Can you work these out from the drawing? Everything is in mm from the part's minimum corner. A direction names the side the tool comes from. Coordinates: 2 decimals unless noted, no trailing zeros. Write each loop counter-clockwise with the first axis right and the second up, starting at its lowest first coordinate (ties: lowest second). Pieces come first, ordered by that corner, then holes. Notation, with made-up numbers: M 13,32.25 L 67,32.25 A27 cw 67,66.25 Z; hole C -13,39 d8. An arc over 180 degrees is marked long. Write item = value, one per line.
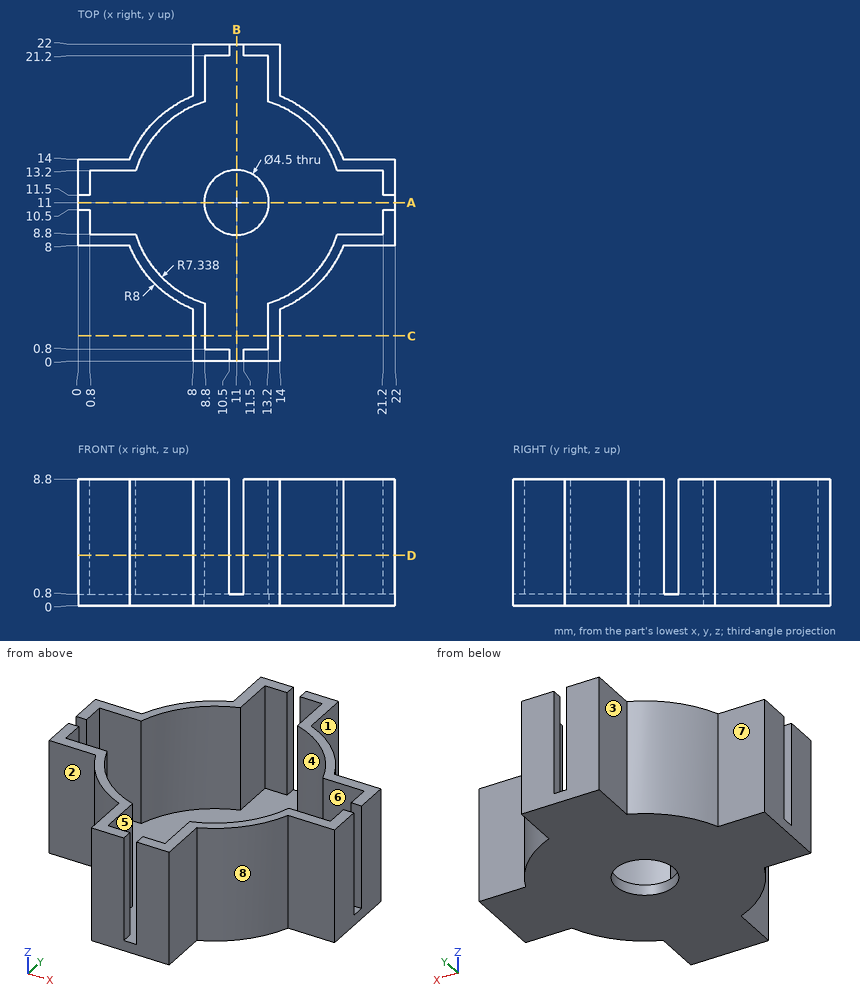
Item 1: I'm going to push flat-ended pins straight in: P1, Ø3.5, axis at y = 19, z = 6, coming from the +X side (1 decimal); P2, Ø1.6, axis at x = 1.5, z = 3, coming from the +Y side; P3, Ø1, axis at x = 3.5, z = 6, coming from the -Y side (1 decimal); P4, Ø1.4, axis at x = 9.5, z = 6, coming from the -Y side. Where does each tip first touch, or does it pass through?
Numbers:
P1 = 16
P2 = 14
P3 = 7.1
P4 = 0
Item 2: Imagine slicing it at D-D (z = 3.5). State how many separate pieces and enclosed holes the cut face has.
Numbers:
separate_pieces = 4
enclosed_holes = 0
Item 3: If I drill on line 1 along X through (y, z) = (18.5, 7); line 2 along Y through (x, z) = (11, 0.2), over which ranges is the centre line in solid material (lowest first)?
Numbers:
line_1 = 8 to 8.8, 13.2 to 14
line_2 = 0 to 8.75, 13.25 to 22
Item 4: Imagine slicing it at C-C (y = 1.75). Write out the boundary of the cut face in (x, z).
Numbers:
outline = M 8,0 L 14,0 L 14,8.8 L 13.2,8.8 L 13.2,0.8 L 8.8,0.8 L 8.8,8.8 L 8,8.8 Z
Item 5: For the marked faces 1, 2, 3 and 4, which set-ups out of +Z, -Z, +X, -X, +Y, -Y let a thin tool reach every point of the face, with its end or its side?
Numbers:
face_1 = +Z, -Z, +X, +Y
face_2 = +Z, -Z, -X, -Y
face_3 = +Z, -Z, -X, +Y
face_4 = +Z
Item 6: Imagine slicing it at A-A (y = 11). Write out the boundary of the cut face in (x, z), and give its area (3 significant figures).
Numbers:
outline = M 0,0 L 8.75,0 L 8.75,0.8 L 0,0.8 Z; M 13.25,0 L 22,0 L 22,0.8 L 13.25,0.8 Z
area = 14.0 mm²
Item 7: If we mould it in two halves opening along X, with no side actions, what happens to the marked faces 5, 6, 7 and 8? For each: pulls with the +X half, pulls with the -X half, needs draft (parallel to the pull), parting line crosses it, or undercut.
Numbers:
face_5 = undercut
face_6 = undercut
face_7 = needs draft
face_8 = pulls with the +X half
